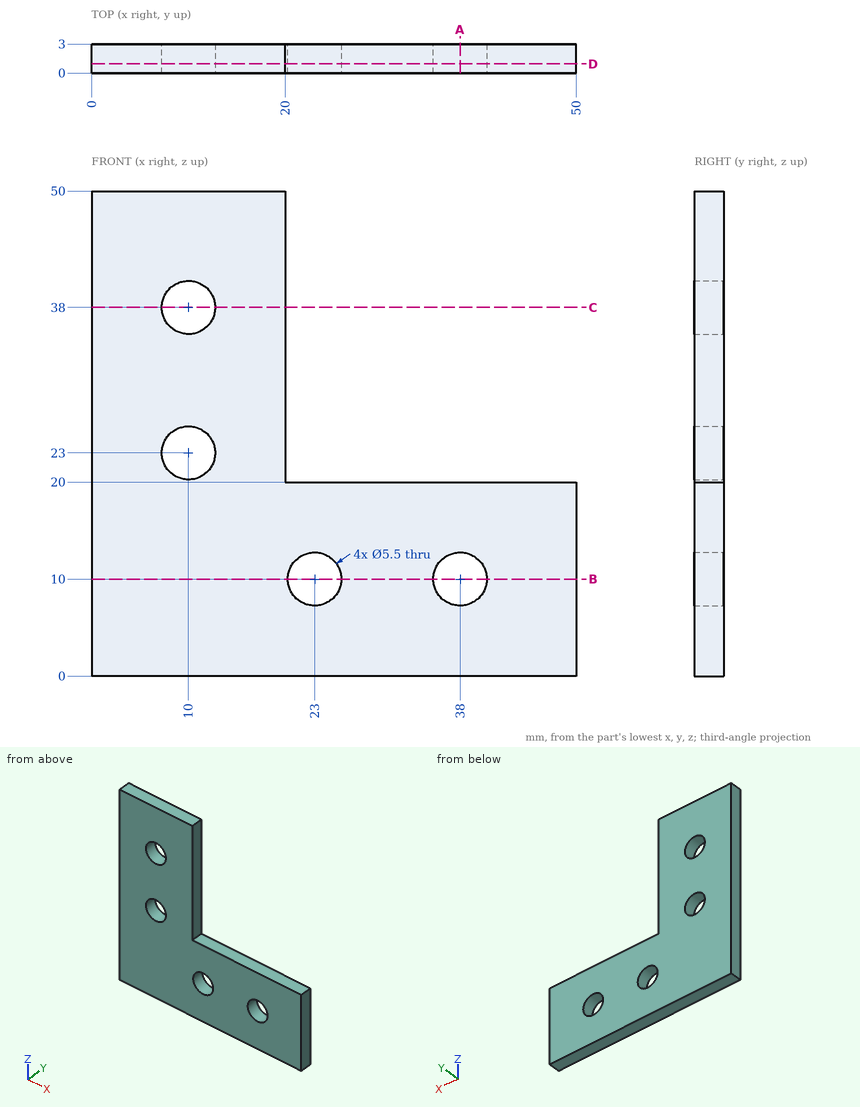
Geometry: see drawing. Coordinates: mm, zero at the bounding-box minimum. Coordinates: 2 decimals unless noted, no trailing zeros. Loops run counter-clockwise (first coordinate to the right, second up) from the corner with the lowest first, then second, coordinate; pieces in that order, holes last.
(1) First-contact query: pin 1 Ø1.5 at (y, z) = (2, 38.5) entering from +X; pin 2 Ø12 at (x, z) = (10.5, 36.5) entering from -Y; pin 3 Ø1.5 at (x, y) = (40.5, 2) entering from +Z. Flat tips, straight axial feed; report the tip coordinate or a pass-through.
(2) Section D-D on y = 0.95. Return the cut outline in (x, z).
(3) Material intervals for probe 1 along Z at (x, y) = (10, 1); probe 2 along X at (y, z) = (1.55, 38), sorted ascending.
(4) Section A-A on x = 38. Return the cut outline in (y, z).
(5) Section B-B on z = 10. Return the cut outline in (x, y), then the cut area to 3 significant figures.
(6) Section C-C on z = 38. Return the cut outline in (x, y), then the cut area to 3 significant figures.
Data:
1. pin 1: stops at x = 20
1. pin 2: stops at y = 0
1. pin 3: stops at z = 20
2. outline: (0, 0) - (50, 0) - (50, 20) - (20, 20) - (20, 50) - (0, 50) - close; hole circle Ø5.5 at (10, 23); hole circle Ø5.5 at (10, 38); hole circle Ø5.5 at (23, 10); hole circle Ø5.5 at (38, 10)
3. probe 1: z = 0 to 20.25, 25.75 to 35.25, 40.75 to 50
3. probe 2: x = 0 to 7.25, 12.75 to 20
4. outline: (0, 0) - (3, 0) - (3, 7.25) - (0, 7.25) - close; (0, 12.75) - (3, 12.75) - (3, 20) - (0, 20) - close
5. outline: (0, 0) - (20.25, 0) - (20.25, 3) - (0, 3) - close; (25.75, 0) - (35.25, 0) - (35.25, 3) - (25.75, 3) - close; (40.75, 0) - (50, 0) - (50, 3) - (40.75, 3) - close
5. area: 117 mm2
6. outline: (0, 0) - (7.25, 0) - (7.25, 3) - (0, 3) - close; (12.75, 0) - (20, 0) - (20, 3) - (12.75, 3) - close
6. area: 43.5 mm2
